The listing builds one solid part. Answer for the finished solid, in the listing's coordinates (mm). Round coordinates to 2 decimals unless told otherwise and drop trailing zeros. Order: outer loops, then holes, each group sorted by start corner. A loop starts at its lowest first (then second) coordinate and runs counter-clockwise, first axis right, second up. Notation, with made-up numbers: (-3.5, 57) - (11.5, 57) arc R6 ccw to (11.5, 62) - close; hole circle Ø9 at (68, -23.75). An arc over 180 degrees is marked (long way). Write item = value, one per line.
from build123d import *

# Parameters (mm, degrees)
SKETCH1_R           = 99
SKETCH1_R_2         = 89
BOSS_EXTRUDE1_DEPTH = 90
FILLET1_R           = 1.5


with BuildPart() as part:
    # Sketch1 → Boss-Extrude1 (new body)
    with BuildSketch(Plane.XY):
        with Locations((232.735026919, 15)):
            Circle(SKETCH1_R)
        with Locations((232.735026919, 15)):
            Circle(SKETCH1_R_2, mode=Mode.SUBTRACT)
    extrude(amount=-BOSS_EXTRUDE1_DEPTH)

    # Fillet1
    fillet1_edges = [part.edges().sort_by_distance(p)[0] for p in [
        (133.735026919, 15, 0),
        (143.735026919, 15, -90),
        (143.735026919, 15, 0),
    ]]
    fillet(fillet1_edges, radius=FILLET1_R)


solid = part.part
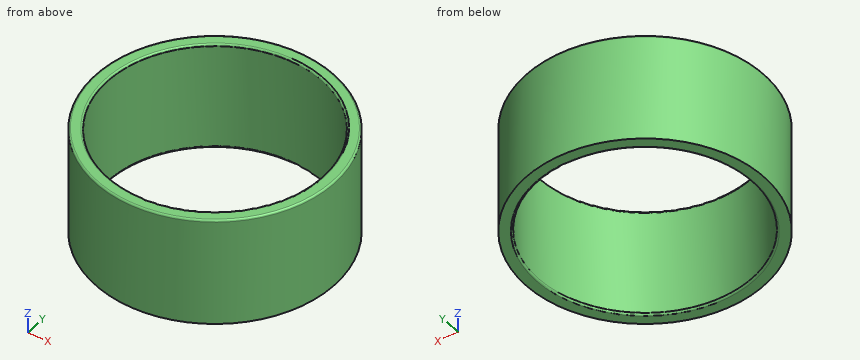
Q1. Section B-B on z = -23 is taken. Determine the outline of the cut face in (x, y), then the cut area to 3 significant figures.
Model answer:
outline = circle Ø198 at (232.74, 15); hole circle Ø178 at (232.74, 15)
area = 5,910 mm^2
Q2. Find the intervals of material crossed by line 1 (Y direction, x = 230, z = -33); line 2 (Y direction, x = 233, z = -66); line 3 (X direction, y = -38, z = -86), in increasing order. Write a range as from..to.
Model answer:
line_1 = -83.96..-73.96, 103.96..113.96
line_2 = -84..-74, 104..114
line_3 = 149.12..161.24, 304.23..316.35
Q3. Section A-A on y = 15 is taken. Determine the outline of the cut face in (x, z), then the cut area to 3 significant figures.
Model answer:
outline = (133.74, -90) - (142.24, -90) arc R1.5 ccw to (143.74, -88.5) - (143.74, -1.5) arc R1.5 ccw to (142.24, 0) - (135.24, 0) arc R1.5 ccw to (133.74, -1.5) - close; (321.74, -88.5) arc R1.5 ccw to (323.24, -90) - (331.74, -90) - (331.74, -1.5) arc R1.5 ccw to (330.24, 0) - (323.24, 0) arc R1.5 ccw to (321.74, -1.5) - close
area = 1,800 mm^2
Q4. Flat-ended cylindrical pins translate along their axes: P1, Ø1.5, axis at x = 255.5, z = -55, coming from the +Y side; P2, Ø1, axis at x = 204, z = -56, coming from the +Y side; P3, Ø12, axis at x = 282.5, z = -11, coming from the +Y side. Find the tip coordinate at first contact, or state that the pin passes through.
Model answer:
P1 = 111.52
P2 = 109.89
P3 = 103.8
